Build history of the part. All positions in model axes, mm. Round coordinates to 2 decimals unless told otherwise and drop trailing zeros. Loops run counter-clockwise (first coordinate to the right, second up) from the corner with the lowest first, then second, coordinate; pieces in that order, holes last. Notation, with made-up numbers: M 64,31.5 L 103,31.5 A6 cw 103,41.5 Z; hole C -17.75,37.5 d10. An arc over 180 degrees is marked long. Use one line per item in the form item = value. Start each with the question number.
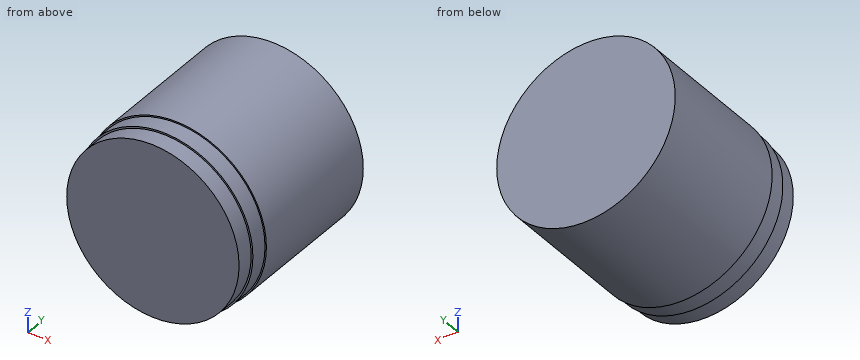
```python
from build123d import *

# Parameters (mm, degrees)
F0_R     = 12.7
F1_DEPTH = 25.4
F2_R     = 12.954
F3_DEPTH = 22.86
F4_R     = 13.1572
F5_DEPTH = 20.32


with BuildPart() as f1:
    # F0 (on Front) → F1 (new body)
    with BuildSketch(Plane.XZ):
        Circle(F0_R)
    extrude(amount=F1_DEPTH)

    # F2 (on Front) → F3 (join)
    with BuildSketch(Plane.XZ):
        Circle(F2_R)
    extrude(amount=F3_DEPTH)

    # F4 (on Front) → F5 (join)
    with BuildSketch(Plane.XZ):
        Circle(F4_R)
    extrude(amount=F5_DEPTH)


solid = f1.part
```
Q1. Drop flat-ended pins along their axis: P1, Ø3, axis at x = 4, y = -16, coming from the +Z side; P2, Ø4, axis at y = -15.5, z = -3, coming from the +X side; P3, Ø2, axis at x = 8, y = -19.5, coming from the +Z side. Give the stop position or say it passes through.
Q2. Saw through at B-B (x = -10.75). Give the cut face in (y, z), and give its area (3 significant figures).
Q3. Saw through at C-C (y = -20.75). Give the cut face in (x, z), and give its area (3 significant figures).
Q4. Saw through at D-D (y = -7.25). Give the cut face in (x, z), and give its area (3 significant figures).
Q5. Saw through at A-A (z = 6). Give the cut face in (x, y), and give its area (3 significant figures).
Q6. Wall check: probe 1 along Z at (x, y) = (0.25, -17.25); probe 2 along Y at (x, z) = (8, -10); probe 3 along Y at (x, z) = (-8.5, -10). Give the ranges that are in metal, low to high.
Filled in:
q1.P1 = 12.92
q1.P2 = 13.12
q1.P3 = 11.14
q2.outline = M -25.4,-6.76 L -22.86,-6.76 L -22.86,-7.23 L -20.32,-7.23 L -20.32,-7.59 L 0,-7.59 L 0,7.59 L -20.32,7.59 L -20.32,7.23 L -22.86,7.23 L -22.86,6.76 L -25.4,6.76 Z
q2.area = 379 mm²
q3.outline = C 0,0 d25.91
q3.area = 527 mm²
q4.outline = C 0,0 d26.31
q4.area = 544 mm²
q5.outline = M -11.71,-20.32 L -11.48,-20.32 L -11.48,-22.86 L -11.19,-22.86 L -11.19,-25.4 L 11.19,-25.4 L 11.19,-22.86 L 11.48,-22.86 L 11.48,-20.32 L 11.71,-20.32 L 11.71,0 L -11.71,0 Z
q5.area = 591 mm²
q6.probe_1 = -13.15 to 13.15
q6.probe_2 = -22.86 to 0
q6.probe_3 = -20.32 to 0
